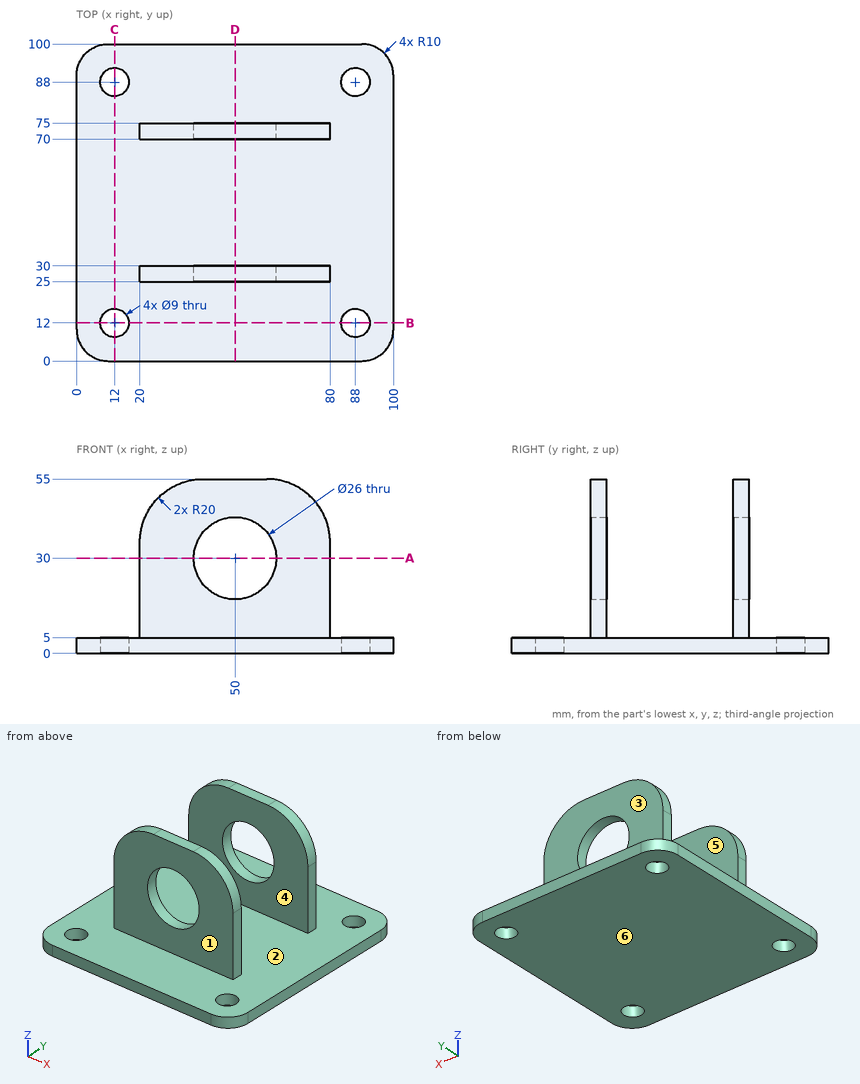
Input: dimensioned drawing with shaded views. Units: mm. Origin: part minimum x, y, z. A direction names the side the tool comes from. Coordinates: 2 decimals unless noted, no trailing zeros. Loops run counter-clockwise (first coordinate to the right, second up) from the corner with the lowest first, then second, coordinate; pieces in that order, holes last. Notation, with made-up numbers: (60.25, -8) -> (88.25, -8) arc R22 ccw to (88.25, 28) -> close; hole circle Ø10 at (-15, 82.5). An arc over 180 degrees is marked (long way). One line per item, written item: value. Start each with the question number.
Q1. Set-up query: the marked faces 5 and 6. Return all of +Z, -Z, +X, -X, +Y, -Y with unobstructed straight access to the full face (end or side cutting, diameter ignored); none if empty.
Q2. Line query: line 1 along Y through (x, z) = (12, 2); line 2 along Y through (x, z) = (35, 24); line 3 along Z through (x, y) = (50, 26.2). Output: solid intervals per line, ascending.
Q3. Section query B-B, the plane y = 12. Return the cut outline in (x, z), and give its area (3 significant figures).
Q4. Mould query, pull axis Y, two halves, no side actions, for the marked faces 1, 2, 3 and 4. Classes: pulls with the +Y half, pulls with the -Y half, needs draft (parallel to the pull), parting line crosses it, or undercut.
Q5. Section query D-D, the plane x = 50. Return the cut outline in (y, z).
Q6. Section query A-A, the plane z = 30. Return the cut outline in (x, y), and give its area (3 significant figures).
Q7. Contact query for flat-ended pins moving along their axis: P1, Ø1.5, axis at y = 27.5, z = 23, coming from the +X side; P2, Ø4, axis at y = 75, z = 47.5, coming from the +X side; P3, Ø6, axis at x = 37, y = 47, coming from the +Z side. Output: stop coordinate, or through.
Results:
1. face 5: +Z, +X, -X
1. face 6: -Z, +X, -X, +Y, -Y
2. line 1: 0 to 7.5, 16.5 to 83.5, 92.5 to 100
2. line 2: 25 to 30, 70 to 75
2. line 3: 0 to 17, 43 to 55
3. outline: (0, 0) -> (7.5, 0) -> (7.5, 5) -> (0, 5) -> close; (16.5, 0) -> (83.5, 0) -> (83.5, 5) -> (16.5, 5) -> close; (92.5, 0) -> (100, 0) -> (100, 5) -> (92.5, 5) -> close
3. area: 410 mm^2
4. face 1: pulls with the -Y half
4. face 2: undercut
4. face 3: pulls with the +Y half
4. face 4: undercut
5. outline: (0, 0) -> (100, 0) -> (100, 5) -> (75, 5) -> (75, 17) -> (70, 17) -> (70, 5) -> (30, 5) -> (30, 17) -> (25, 17) -> (25, 5) -> (0, 5) -> close; (25, 43) -> (30, 43) -> (30, 55) -> (25, 55) -> close; (70, 43) -> (75, 43) -> (75, 55) -> (70, 55) -> close
6. outline: (20, 25) -> (37, 25) -> (37, 30) -> (20, 30) -> close; (20, 70) -> (37, 70) -> (37, 75) -> (20, 75) -> close; (63, 25) -> (80, 25) -> (80, 30) -> (63, 30) -> close; (63, 70) -> (80, 70) -> (80, 75) -> (63, 75) -> close
6. area: 340 mm^2
7. P1: x = 80
7. P2: x = 77.02
7. P3: z = 5
